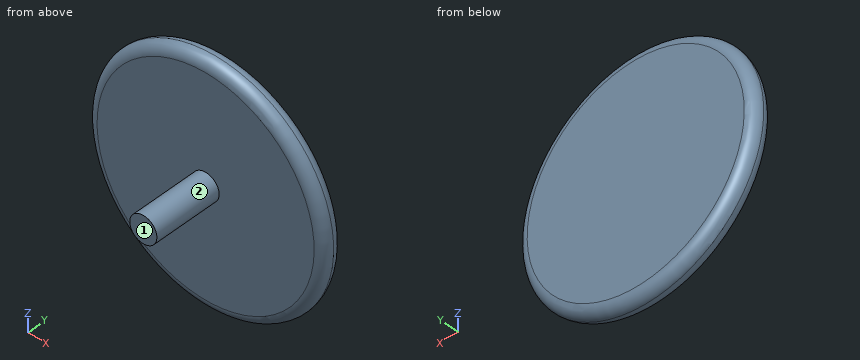
```python
from build123d import *

# Parameters (mm, degrees)
SKETCH1_R           = 2
BOSS_EXTRUDE1_DEPTH = 10
SKETCH2_R           = 17.5
BOSS_EXTRUDE2_DEPTH = 3
FILLET1_R           = 1.5


with BuildPart() as part:
    # Sketch1 → Boss-Extrude1 (new body)
    with BuildSketch(Plane(origin=(0, 0, 0), x_dir=(1, 0, 0), z_dir=(0, 1, 0))):
        with Locations(Location((0, 0, 0), (0, 0, 270))):
            Circle(SKETCH1_R)
    extrude(amount=BOSS_EXTRUDE1_DEPTH)

    # Sketch2 → Boss-Extrude2 (add)
    with BuildSketch(Plane(origin=(0, 10, 0), x_dir=(1, 0, 0), z_dir=(0, 1, 0))):
        with Locations(Location((0, 0, 0), (0, 0, 270))):
            Circle(SKETCH2_R)
    extrude(amount=BOSS_EXTRUDE2_DEPTH)

    # Fillet1
    fillet1_edges = [part.edges().sort_by_distance(p)[0] for p in [
        (0, 10, -17.5),
        (0, 13, -17.5),
    ]]
    fillet(fillet1_edges, radius=FILLET1_R - 0.0001)  # a hair under: the kernel refuses the full size


solid = part.part
```
Design review of the part built by this model. Coordinates are the model's own, in mm. Face numbers are marked on the shaded views. A direction names the side the tool comes from. Give positions to 0.01 mm unless a question says otherwise; leave off trailing zeros. Order: outer loops, then holes, each group sorted by start corner. A loop starts at its lowest first (then second) coordinate and runs counter-clockwise, first axis right, second up. Notation, with made-up numbers: (57, -14.5) - (103, -14.5) arc R21 cw to (103, 11.5) - close; hole circle Ø1 at (43, 11). An arc over 180 degrees is marked (long way). Use a Markdown table: item, result. Add a question column.
(1) Clearance check with flat-ended pins moving along their axes: P1, Ø6, axis at x = -4.5, y = 3.5, coming from the -Z side; P2, Ø1.5, axis at x = 2, y = 4, coming from the -Z side; P3, Ø2, axis at x = -12, z = -10.5, coming from the -Y side. State where each tip first meets the part, or that it passes through.
(2) Add section C-C on y = 4. Give the boundary of the cut face in (x, z).
(3) Wall thickness on probe 1 along Y at (x, z) = (11, 5); probe 2 along X at (y, z) = (5, -1.5); probe 3 along Z at (x, y) = (-15, 10.5): over which ranges is each line inside the solid? List them lowest first. Write a range as [from, to].
(4) Machinability: for the marked faces 1 and 2, which of the approach directions +Z, -Z, +X, -X, +Y, -Y give a long, thin tool a straight path to every point of the face, cutting with its end or side? Answer none if there is none.
Report:
| question | item | result |
|---|---|---|
| 1 | P1 | stops at z = -1.32 |
| 1 | P2 | stops at z = -1.56 |
| 1 | P3 | stops at y = 10 |
| 2 | outline | circle Ø4 at (0, 0) |
| 3 | probe 1 | y = [10, 13] |
| 3 | probe 2 | x = [-1.32, 1.32] |
| 3 | probe 3 | z = [-8.25, 8.25] |
| 4 | face 1 | +Z, -Z, +X, -X, -Y |
| 4 | face 2 | -Y |
